Input: part model. Units: mm. Frame: model coordinates. Round coordinates to 2 decimals unless told otherwise and drop trailing zeros. Order: outer loops, then holes, each group sorted by start corner. A loop starts at its lowest first (then second) coordinate and runs counter-clockwise, first axis right, second up. Notation, with made-up numbers: (57, -1) -> (116, -1) arc R21 cw to (116, 15) -> close; hole circle Ø2 at (48.25, 46.5). An arc over 180 degrees is marked (long way). Answer as CSV lines item,"result". Start each with the question number.
1) Line query: L1, parallel to Y at x = 0, z = 2.75; L2, parallel to Y at x = 5, z = 4.25; L3, parallel to X at y = -25.5, z = 1.25. Output: solid intervals per line, ascending.
2) First-contact query: P1, Ø2, axis at x = 9, z = 5, coming from the +Y side. Flat tip, straight axial feed; report the tip coordinate or a pass-through.
3) Section query C-C, the plane z = 2.75. Output: boundary loops of the cut face in (x, y).
4) Section query D-D, the plane y = -18.5. Output: boundary loops of the cut face in (x, z).
5) Section query A-A, the plane y = 0. Output: boundary loops of the cut face in (x, z), and give its area (3 significant figures).
6) Section query B-B, the plane x = 0. Output: boundary loops of the cut face in (y, z), and give its area (3 significant figures).
7) Mould query, pull axis Y, two halves, no side actions, for faces 1 (the face through (-2.406, 14.164, 3.451)), 2 (the face through (12.5, 0, 3)), 3 (the face through (0, -37.5, 3)). Classes: +Y half, -Y half, draft (parallel to the pull), parting line (faces both ways), or undercut.
```python
from build123d import *

# Parameters (mm, degrees)
F0_R     = 11.1
F1_DEPTH = 7
F2_R     = 5


with BuildPart() as f1:
    # F0 (on Top) → F1 (new body)
    with BuildSketch(Plane.XY):
        Polygon((12.5, 25), (12.5, 37.5), (-12.5, 37.5), (-12.5, 25), (-12.5, 12.5), (-12.5, -12.5), (-12.5, -25), (-12.5, -37.5), (12.5, -37.5), (12.5, -25), (12.5, -12.5), (12.5, 12.5), align=None)
        with Locations((0, -25)):
            Circle(F0_R, mode=Mode.SUBTRACT)
        Circle(F0_R, mode=Mode.SUBTRACT)
        with Locations((0, 25)):
            Circle(F0_R, mode=Mode.SUBTRACT)
    extrude(amount=F1_DEPTH)

    # F2
    f2_edges = [f1.edges().sort_by_distance(p)[0] for p in [
        (12.5, -37.5, 3.5),
        (-12.5, -37.5, 3.5),
        (-12.5, 37.5, 3.5),
        (12.5, 37.5, 3.5),
    ]]
    fillet(f2_edges, radius=F2_R)


solid = f1.part
```
Findings:
1,L1,"y = -37.5 to -36.1, -13.9 to -11.1, 11.1 to 13.9, 36.1 to 37.5"
1,L2,"y = -37.5 to -34.91, -15.09 to -9.91, 9.91 to 15.09, 34.91 to 37.5"
1,L3,"x = -12.5 to -11.09, 11.09 to 12.5"
2,P1,"stops at y = 37.47"
3,outline,"(-12.5, -32.5) arc R5 ccw to (-7.5, -37.5) -> (7.5, -37.5) arc R5 ccw to (12.5, -32.5) -> (12.5, 32.5) arc R5 ccw to (7.5, 37.5) -> (-7.5, 37.5) arc R5 ccw to (-12.5, 32.5) -> close; hole circle Ø22.2 at (0, -25); hole circle Ø22.2 at (0, 0); hole circle Ø22.2 at (0, 25)"
4,outline,"(-12.5, 0) -> (-9, 0) -> (-9, 7) -> (-12.5, 7) -> close; (9, 0) -> (12.5, 0) -> (12.5, 7) -> (9, 7) -> close"
5,outline,"(-12.5, 0) -> (-11.1, 0) -> (-11.1, 7) -> (-12.5, 7) -> close; (11.1, 0) -> (12.5, 0) -> (12.5, 7) -> (11.1, 7) -> close"
5,area,"19.6 mm^2"
6,outline,"(-37.5, 0) -> (-36.1, 0) -> (-36.1, 7) -> (-37.5, 7) -> close; (-13.9, 0) -> (-11.1, 0) -> (-11.1, 7) -> (-13.9, 7) -> close; (11.1, 0) -> (13.9, 0) -> (13.9, 7) -> (11.1, 7) -> close; (36.1, 0) -> (37.5, 0) -> (37.5, 7) -> (36.1, 7) -> close"
6,area,"58.8 mm^2"
7,face 1,"undercut"
7,face 2,"draft"
7,face 3,"-Y half"
